For this review, use the dimensioned drawing (mm, ordinates from the lowest corner) and the shaded views. Give positions to 0.01 mm unless a question says otherwise; leave off trailing zeros. Write each loop counter-clockwise with the first axis right and the second up, starting at its lowest first coordinate (ties: lowest second). Pieces come first, ordered by that corner, then holes. Notation, with made-up numbers: (-7, 63.5) -> (29, 63.5) arc R30 ccw to (29, 99.5) -> close; hole circle Ø10 at (14, 48.25). An arc over 180 degrees is marked (long way). Answer as CSV lines item,"result".
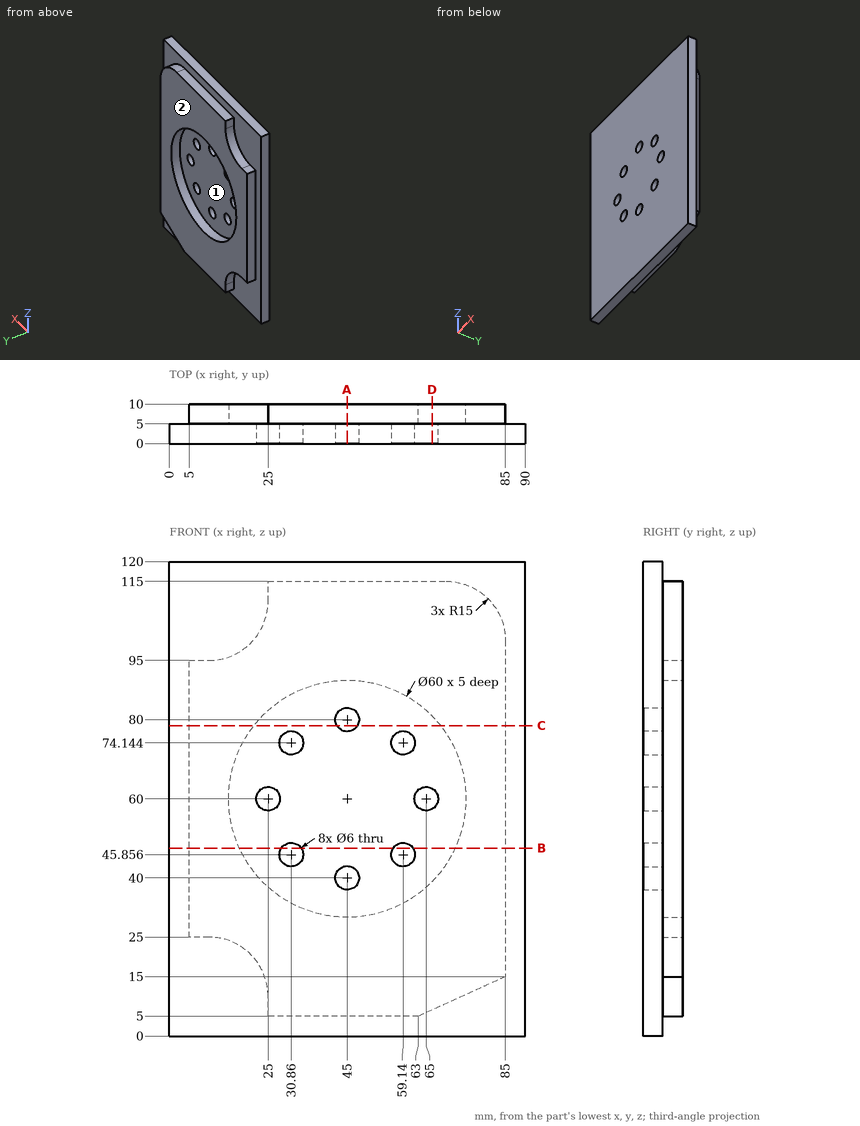
Q1. Add section A-A (x = 45). Write out the cut boundary in (y, z).
Answer block:
outline,"(0, 0) -> (5, 0) -> (5, 5) -> (10, 5) -> (10, 30) -> (5, 30) -> (5, 37) -> (0, 37) -> close; (0, 43) -> (5, 43) -> (5, 77) -> (0, 77) -> close; (0, 83) -> (5, 83) -> (5, 90) -> (10, 90) -> (10, 115) -> (5, 115) -> (5, 120) -> (0, 120) -> close"
Q2. Add section B-B (z = 47.5). Write out the cut boundary in (x, y).
Answer block:
outline,"(0, 0) -> (28.35, 0) -> (28.35, 5) -> (17.73, 5) -> (17.73, 10) -> (5, 10) -> (5, 5) -> (0, 5) -> close; (33.37, 0) -> (56.63, 0) -> (56.63, 5) -> (33.37, 5) -> close; (61.65, 0) -> (90, 0) -> (90, 5) -> (85, 5) -> (85, 10) -> (72.27, 10) -> (72.27, 5) -> (61.65, 5) -> close"
Q3. Add section C-C (z = 78.5). Write out the cut boundary in (x, y), plus the area to 3 significant figures.
Answer block:
outline,"(0, 0) -> (42.4, 0) -> (42.4, 5) -> (21.38, 5) -> (21.38, 10) -> (5, 10) -> (5, 5) -> (0, 5) -> close; (47.6, 0) -> (90, 0) -> (90, 5) -> (85, 5) -> (85, 10) -> (68.62, 10) -> (68.62, 5) -> (47.6, 5) -> close"
area,"588 mm2"
Q4. Clearance check with flat-ended pins moving along their axes: pin 1 (1.5 mm diameter, centred on y = 6, z = 67, fed in from -X); pin 2 (10 mm diameter, centred on x = 60, z = 62, fed in from +Y); pin 3 (9.5 mm diameter, centred on x = 30.86, z = 74.14, fed in from -Y); pin 4 (5 mm diameter, centred on x = 45, z = 80, fed in from +Y). State where each tip first meets the part, or that it passes through.
Answer block:
pin 1,"stops at x = 5"
pin 2,"stops at y = 5"
pin 3,"stops at y = 0"
pin 4,"passes through"
Q5. To check wall thickness, follow probe 1 along Z at (x, y) = (30.86, 3.95); probe 2 along Z at (x, y) = (25, 1.8); probe 3 along Z at (x, y) = (46, 6.5). State the ranges of each line that lie inside material, in increasing order. Write a range as [from, to].
Answer block:
probe 1,"z = [0, 42.86], [48.86, 71.14], [77.14, 120]"
probe 2,"z = [0, 57], [63, 120]"
probe 3,"z = [5, 30.02], [89.98, 115]"
Q6. Add section D-D (x = 66.5). Write out the cut boundary in (y, z), plus the area to 3 significant figures.
Answer block:
outline,"(0, 0) -> (5, 0) -> (5, 6.59) -> (10, 6.59) -> (10, 39.08) -> (5, 39.08) -> (5, 57.4) -> (0, 57.4) -> close; (0, 62.6) -> (5, 62.6) -> (5, 80.92) -> (10, 80.92) -> (10, 115) -> (5, 115) -> (5, 120) -> (0, 120) -> close"
area,"907 mm2"
Q7. Draft analysis for pull direction X (two halves, no side actions). For the marked faces 1 and 2, state which applies: released by +X, released by -X, zero draft, split by the parting line, or undercut.
Answer block:
face 1,"undercut"
face 2,"zero draft"
